from build123d import *

# Parameters (mm, degrees)
SKETCH1_W           = 71
SKETCH1_H           = 34
BOSS_EXTRUDE1_DEPTH = 7
SHELL1_T            = -2.4
SKETCH3_W           = 17
SKETCH3_H           = 34
BOSS_EXTRUDE2_DEPTH = 7
SKETCH4_W           = 14.6
SKETCH4_H           = 29.2
CUT_EXTRUDE2_DEPTH  = 4.6
SKETCH5_W           = 19.3
SKETCH5_H           = 0.4
CUT_EXTRUDE3_DEPTH  = 4.6
CUT_EXTRUDE4_DEPTH  = 2
SKETCH7_W           = 17.3
SKETCH7_H           = 7.4
BOSS_EXTRUDE3_DEPTH = 4.6
FILLET1_R           = 3
SKETCH8_R           = 2.5546875
BOSS_EXTRUDE4_DEPTH = 7
CUT_EXTRUDE5_REACH  = 57.626
SKETCH9_R           = 1.25
SKETCH10_R          = 2.15
CUT_EXTRUDE6_DEPTH  = 1.6


with BuildPart() as part:
    # Sketch1 → Boss-Extrude1 (new body)
    with BuildSketch(Plane(origin=(0, 0, 0), x_dir=(1, 0, 0), z_dir=(0, 1, 0))):
        Rectangle(SKETCH1_W, SKETCH1_H)
    extrude(amount=BOSS_EXTRUDE1_DEPTH)

    # Shell1
    shell1_openings = [part.faces().sort_by_distance(p)[0] for p in [
        (0, 7, 0),
    ]]
    offset(amount=SHELL1_T, openings=shell1_openings, kind=Kind.INTERSECTION)

    # Sketch3 → Boss-Extrude2 (add)
    with BuildSketch(Plane.XZ):
        with Locations((44, 0)):
            Rectangle(SKETCH3_W, SKETCH3_H)
    extrude(amount=-BOSS_EXTRUDE2_DEPTH)

    # Sketch4 → Cut-Extrude2 (cut)
    with BuildSketch(Plane(origin=(0, 7, 0), x_dir=(1, 0, 0), z_dir=(0, 1, 0))):
        with Locations((42.8, 0)):
            Rectangle(SKETCH4_W, SKETCH4_H)
    extrude(amount=-CUT_EXTRUDE2_DEPTH, mode=Mode.SUBTRACT)

    # Sketch5 → Cut-Extrude3 (cut)
    with BuildSketch(Plane(origin=(0, 7, 0), x_dir=(1, 0, 0), z_dir=(0, 1, 0))):
        with Locations((20, -14.8)):
            Rectangle(SKETCH5_W, SKETCH5_H)
    extrude(amount=-CUT_EXTRUDE3_DEPTH, mode=Mode.SUBTRACT)

    # Sketch6 → Cut-Extrude4 (cut)
    with BuildSketch(Plane.XY.offset(17)):
        Polygon((16.1, 4.737867966), (16.987867966, 3.85), (23.012132034, 3.85), (23.9, 4.737867966), (23.9, 6.3), (23.9, 7), (16.1, 7), (16.1, 6.3), align=None)
    extrude(amount=-CUT_EXTRUDE4_DEPTH, mode=Mode.SUBTRACT)

    # Sketch7 → Boss-Extrude3 (add)
    with BuildSketch(Plane(origin=(0, 2.4, 0), x_dir=(1, 0, 0), z_dir=(0, 1, 0))):
        with Locations((20, 10.9)):
            Rectangle(SKETCH7_W, SKETCH7_H)
    extrude(amount=BOSS_EXTRUDE3_DEPTH)

    # Fillet1
    fillet1_edges = [part.edges().sort_by_distance(p)[0] for p in [
        (52.5, 3.5, -17),
        (52.5, 3.5, 17),
        (-35.5, 3.5, 17),
        (-35.5, 3.5, -17),
    ]]
    fillet(fillet1_edges, radius=FILLET1_R)

    # Sketch8 → Boss-Extrude4 (add)
    with BuildSketch(Plane(origin=(0, 0, 0), x_dir=(-1, 0, 0), z_dir=(0, -1, 0))):
        with Locations((32.5, 14)):
            Circle(SKETCH8_R)
        with Locations((32.5, -14)):
            Circle(SKETCH8_R)
        with Locations((-34.3, 14)):
            Circle(SKETCH8_R)
        with Locations((-34.3, -14)):
            Circle(SKETCH8_R)
    extrude(amount=-BOSS_EXTRUDE4_DEPTH)

    # Sketch9 → Cut-Extrude5 (cut, up to next)
    with BuildSketch(Plane.XZ, mode=Mode.PRIVATE) as cut_extrude5_sk1:
        with Locations(Location((-32.5, -14, 0), (0, 0, 270))):
            Circle(SKETCH9_R)
    cut_extrude5_tool1 = extrude(cut_extrude5_sk1.sketch, amount=-CUT_EXTRUDE5_REACH, mode=Mode.PRIVATE) & part.part
    # Sketch9 → Cut-Extrude5 (cut, up to next)
    with BuildSketch(Plane.XZ, mode=Mode.PRIVATE) as cut_extrude5_sk2:
        with Locations(Location((-32.5, 14, 0), (0, 0, 270))):
            Circle(SKETCH9_R)
    cut_extrude5_tool2 = extrude(cut_extrude5_sk2.sketch, amount=-CUT_EXTRUDE5_REACH, mode=Mode.PRIVATE) & part.part
    # Sketch9 → Cut-Extrude5 (cut, up to next)
    with BuildSketch(Plane.XZ, mode=Mode.PRIVATE) as cut_extrude5_sk3:
        with Locations(Location((34.3, -14, 0), (0, 0, 270))):
            Circle(SKETCH9_R)
    cut_extrude5_tool3 = extrude(cut_extrude5_sk3.sketch, amount=-CUT_EXTRUDE5_REACH, mode=Mode.PRIVATE) & part.part
    # Sketch9 → Cut-Extrude5 (cut, up to next)
    with BuildSketch(Plane.XZ, mode=Mode.PRIVATE) as cut_extrude5_sk4:
        with Locations(Location((34.3, 14, 0), (0, 0, 270))):
            Circle(SKETCH9_R)
    cut_extrude5_tool4 = extrude(cut_extrude5_sk4.sketch, amount=-CUT_EXTRUDE5_REACH, mode=Mode.PRIVATE) & part.part
    add(cut_extrude5_tool1.solids().sort_by_distance((-32.5, 0, -14))[0], mode=Mode.SUBTRACT)
    add(cut_extrude5_tool2.solids().sort_by_distance((-32.5, 0, 14))[0], mode=Mode.SUBTRACT)
    add(cut_extrude5_tool3.solids().sort_by_distance((34.3, 0, -14))[0], mode=Mode.SUBTRACT)
    add(cut_extrude5_tool4.solids().sort_by_distance((34.3, 0, 14))[0], mode=Mode.SUBTRACT)

    # Sketch10 → Cut-Extrude6 (cut)
    with BuildSketch(Plane.XZ):
        with Locations(Location((34.3, 14, 0), (0, 0, 270))):
            Circle(SKETCH10_R)
        with Locations(Location((-32.5, -14, 0), (0, 0, 270))):
            Circle(SKETCH10_R)
        with Locations(Location((-32.5, 14, 0), (0, 0, 270))):
            Circle(SKETCH10_R)
        with Locations(Location((34.3, -14, 0), (0, 0, 270))):
            Circle(SKETCH10_R)
    extrude(amount=-CUT_EXTRUDE6_DEPTH, mode=Mode.SUBTRACT)


solid = part.part
Check sheet for the modelled part. Datum: model origin and axes. Units: mm. A direction names the side the tool comes from. Give positions to 0.01 mm unless a question says otherwise; leave off trailing zeros. Loops run counter-clockwise (first coordinate to the right, second up) from the corner with the lowest first, then second, coordinate; pieces in that order, holes last. Notation, with made-up numbers: M 10,24.5 L 19,24.5 A17 cw 19,45.5 Z; hole C 21.5,27 d5. An arc over 180 degrees is marked long. Use a Markdown table: item, result. Add a question column.
Q1. Scan lines: line 1 along X through (y, z) = (4, 5); line 2 along X through (y, z) = (0.55, -14); line 3 along X through (y, z) = (3.45, 14). Record each from-to range of solid material in increasing order. Write a range as [from, to].
Q2. Sectioned sample at C-C, the plane x = -2. Record the cut outline in (y, z), then the cut area to 3 significant figures.
Q3. Tool access check on faces 4 (the cylindrical face through (-31.655, 4.262, 14.921)), 5 (the flat face through (20, 3.85, 16)), 6 (the flat face through (-32.5, 1.6, 12.6)), 7 (the flat face through (35.5, 5, 0)). Record the directions out of +Z, -Z, +X, -X, +Y, -Y that give a thin tool (end or side, any length) a straight path to the whole face; none if there is none.
Q4. Sectioned sample at B-B, the plane z = 5. Record the cut outline in (x, y), then the cut area to 3 significant figures.
Q5. Sectioned sample at A-A, the plane x = 34.3. Record the cut outline in (y, z), then the cut area to 3 significant figures.
Q6. Sectioned sample at D-D, the plane y = 6. Give the number of separate pieces and of enclosed holes in the cut face, then the cut area to 3 significant figures.
Q7. Mould release check, pull along Z, two halves, no side actions. Record for faces 1 (the flat face through (16.1, 6, 16)), 2 (the cylindrical face through (-34.6, 3.55, -16.14)), 3 (the flat face through (33, 1.6, 13)): pulls with the +Z half, pulls with the -Z half, needs draft (parallel to the pull), parting line crosses it, or undercut.
Q8. Go/stop test with flat-tipped pins: pin 1 (4.5 mm diameter, centred on x = 35, z = 13.5, fed in from -Y); pin 2 (1.5 mm diameter, centred on x = 30.5, z = 10.5, fed in from +Y); pin 3 (1.3 mm diameter, centred on x = -33, z = 14, fed in from -Y); pin 4 (3 mm diameter, centred on x = 34.3, z = -14, fed in from -Y). Record where each tip stops, or that it passes through.
Verdict:
| question | item | result |
|---|---|---|
| 1 | line 1 | [-35.5, -33.1], [33.1, 35.5], [50.1, 52.5] |
| 1 | line 2 | [-35.5, -34.65], [-30.35, 32.15], [36.45, 52.5] |
| 1 | line 3 | [-35.5, -33.75], [-31.25, -29.95], [31.75, 33.05], [35.55, 36.85], [50.1, 52.5] |
| 2 | outline | M 0,-17 L 7,-17 L 7,-14.6 L 2.4,-14.6 L 2.4,14.6 L 7,14.6 L 7,17 L 0,17 Z |
| 2 | area | 104 mm^2 |
| 3 | face 4 | +Y, -Y |
| 3 | face 5 | +Z, +Y |
| 3 | face 6 | -Y |
| 3 | face 7 | +Y |
| 4 | outline | M -35.5,0 L 52.5,0 L 52.5,7 L 50.1,7 L 50.1,2.4 L 35.5,2.4 L 35.5,7 L 33.1,7 L 33.1,2.4 L -33.1,2.4 L -33.1,7 L -35.5,7 Z |
| 4 | area | 244 mm^2 |
| 5 | outline | M 0,-17 L 7,-17 L 7,-15.25 L 1.6,-15.25 L 1.6,-16.15 L 0,-16.15 Z; M 0,-11.85 L 1.6,-11.85 L 1.6,-12.75 L 7,-12.75 L 7,12.75 L 1.6,12.75 L 1.6,11.85 L 0,11.85 Z; M 0,16.15 L 1.6,16.15 L 1.6,15.25 L 7,15.25 L 7,17 L 0,17 Z |
| 5 | area | 197 mm^2 |
| 6 | separate pieces | 1 |
| 6 | enclosed holes | 5 |
| 6 | area | 739 mm^2 |
| 7 | face 1 | needs draft |
| 7 | face 2 | pulls with the -Z half |
| 7 | face 3 | undercut |
| 8 | pin 1 | y = 0 |
| 8 | pin 2 | y = 2.4 |
| 8 | pin 3 | through |
| 8 | pin 4 | y = 1.6 |
